Here's how the part is built. I have some questions about the finished solid (model axes, mm). Face numbers are marked on the shaded views. A direction names the side the tool comes from. Coordinates: 2 decimals unless noted, no trailing zeros. Loops run counter-clockwise (first coordinate to the right, second up) from the corner with the lowest first, then second, coordinate; pieces in that order, holes last.
from build123d import *

# Parameters (mm, degrees)
F0_R     = 5
F0_R_2   = 3.15
F0_R_3   = 2.55
F1_DEPTH = 3.25
F2_R     = 2.55
F3_DEPTH = 14


# Not quite as in the source:
# - a feature names something its author has since deleted; it is built from what else it names


with BuildPart() as f1:
    # F0 (on Top) → F1 (new body)
    with BuildSketch(Plane.XY):
        with BuildLine():
            Line((-5.95, -4.4), (-4.4034787385, -4.4))
            ThreePointArc((-4.4034787385, -4.4), (0, -6.225), (4.4034787385, -4.4))
            Line((4.4034787385, -4.4), (5.95, -4.4))
            Line((5.95, -4.4), (5.95, 4.4))
            Line((5.95, 4.4), (4.4034787385, 4.4))
            ThreePointArc((4.4034787385, 4.4), (0, 6.225), (-4.4034787385, 4.4))
            Line((-4.4034787385, 4.4), (-5.95, 4.4))
            Line((-5.95, 4.4), (-5.95, -4.4))
        make_face()
        Circle(F0_R, mode=Mode.SUBTRACT)
        Circle(F0_R)
        Circle(F0_R_2, mode=Mode.SUBTRACT)
        Circle(F0_R_2)
        Circle(F0_R_3, mode=Mode.SUBTRACT)
        Circle(F0_R_3)
        with BuildLine():
            ThreePointArc((-1.275, -0.9666307465), (-0.5099019514, 1.5165750888), (1.6, 0))
            ThreePointArc((1.6, 0), (1.5165750888, -0.5099019514), (1.275, -0.9666307465))
            ThreePointArc((1.275, -0.9666307465), (0, -1.6), (-1.275, -0.9666307465))
        make_face(mode=Mode.SUBTRACT)
        with BuildLine():
            Line((1.275, -0.9666307465), (-1.275, -0.9666307465))
            ThreePointArc((-1.275, -0.9666307465), (0, -1.6), (1.275, -0.9666307465))
        make_face()
    extrude(amount=F1_DEPTH)

    # F2 (on face) → F3 (join)
    with BuildSketch(Plane.XY.offset(3.25)):
        with BuildLine():
            ThreePointArc((-4.8302633262, 0.3000085552), (-4.9546244936, 0.172348246), (-5, 0))
            ThreePointArc((-5, 0), (-4.9546244936, -0.172348246), (-4.8302633262, -0.3000085552))
            Line((-4.8302633262, -0.3000085552), (-4.2601369618, -0.6425750355))
            ThreePointArc((-4.2601369618, -0.6425750355), (-4.0929165173, -0.7205512094), (-3.9131380826, -0.7620563314))
            Line((-3.9131380826, -0.7620563314), (-3.3117988826, -0.835891501))
            ThreePointArc((-3.3117988826, -0.835891501), (-3.0868883315, -0.9291389359), (-2.9422567869, -1.125))
            ThreePointArc((-2.9422567869, -1.125), (-3.15, 0), (-2.9422567869, 1.125))
            ThreePointArc((-2.9422567869, 1.125), (-3.0868883315, 0.9291389359), (-3.3117988826, 0.835891501))
            Line((-3.3117988826, 0.835891501), (-3.9131380826, 0.7620563314))
            ThreePointArc((-3.9131380826, 0.7620563314), (-4.0929165173, 0.7205512094), (-4.2601369618, 0.6425750355))
            Line((-4.2601369618, 0.6425750355), (-4.8302633262, 0.3000085552))
        make_face()
        with BuildLine():
            ThreePointArc((-3.2033738691, 3.6276500367), (-3.3815799641, 3.6253171911), (-3.5355339059, 3.5355339059))
            ThreePointArc((-3.5355339059, 3.5355339059), (-3.6253171911, 3.3815799641), (-3.6276500367, 3.2033738691))
            Line((-3.6276500367, 3.2033738691), (-3.4667408995, 2.5580025694))
            ThreePointArc((-3.4667408995, 2.5580025694), (-3.4036356706, 2.3846223779), (-3.3058616735, 2.2281512744))
            Line((-3.3058616735, 2.2281512744), (-2.9328599965, 1.7507308991))
            ThreePointArc((-2.9328599965, 1.7507308991), (-2.8397601142, 1.5257592297), (-2.8759848548, 1.2849945972))
            ThreePointArc((-2.8759848548, 1.2849945972), (-2.2273863607, 2.2273863607), (-1.2849945972, 2.8759848548))
            ThreePointArc((-1.2849945972, 2.8759848548), (-1.5257592297, 2.8397601142), (-1.7507308991, 2.9328599965))
            Line((-1.7507308991, 2.9328599965), (-2.2281512744, 3.3058616735))
            ThreePointArc((-2.2281512744, 3.3058616735), (-2.3846223779, 3.4036356706), (-2.5580025694, 3.4667408995))
            Line((-2.5580025694, 3.4667408995), (-3.2033738691, 3.6276500367))
        make_face()
        with BuildLine():
            ThreePointArc((0.3000085552, 4.8302633262), (0.172348246, 4.9546244936), (0, 5))
            ThreePointArc((0, 5), (-0.172348246, 4.9546244936), (-0.3000085552, 4.8302633262))
            Line((-0.3000085552, 4.8302633262), (-0.6425750355, 4.2601369618))
            ThreePointArc((-0.6425750355, 4.2601369618), (-0.7205512094, 4.0929165173), (-0.7620563314, 3.9131380826))
            Line((-0.7620563314, 3.9131380826), (-0.835891501, 3.3117988826))
            ThreePointArc((-0.835891501, 3.3117988826), (-0.9291389359, 3.0868883315), (-1.125, 2.9422567869))
            ThreePointArc((-1.125, 2.9422567869), (0, 3.15), (1.125, 2.9422567869))
            ThreePointArc((1.125, 2.9422567869), (0.9291389359, 3.0868883315), (0.835891501, 3.3117988826))
            Line((0.835891501, 3.3117988826), (0.7620563314, 3.9131380826))
            ThreePointArc((0.7620563314, 3.9131380826), (0.7205512094, 4.0929165173), (0.6425750355, 4.2601369618))
            Line((0.6425750355, 4.2601369618), (0.3000085552, 4.8302633262))
        make_face()
        with BuildLine():
            ThreePointArc((3.2033738691, -3.6276500367), (3.3815799667, -3.6253171904), (3.5355339096, -3.5355339023))
            ThreePointArc((3.5355339096, -3.5355339023), (3.6253171918, -3.3815799616), (3.6276500367, -3.2033738691))
            Line((3.6276500367, -3.2033738691), (3.4667408995, -2.5580025694))
            ThreePointArc((3.4667408995, -2.5580025694), (3.4036356706, -2.3846223779), (3.3058616735, -2.2281512744))
            Line((3.3058616735, -2.2281512744), (2.9328599965, -1.7507308991))
            ThreePointArc((2.9328599965, -1.7507308991), (2.8397601142, -1.5257592297), (2.8759848548, -1.2849945972))
            ThreePointArc((2.8759848548, -1.2849945972), (2.2273863607, -2.2273863607), (1.2849945972, -2.8759848548))
            ThreePointArc((1.2849945972, -2.8759848548), (1.5257592297, -2.8397601142), (1.7507308991, -2.9328599965))
            Line((1.7507308991, -2.9328599965), (2.2281512744, -3.3058616735))
            ThreePointArc((2.2281512744, -3.3058616735), (2.3846223779, -3.4036356706), (2.5580025694, -3.4667408995))
            Line((2.5580025694, -3.4667408995), (3.2033738691, -3.6276500367))
        make_face()
        with BuildLine():
            ThreePointArc((-0.3000085552, -4.8302633262), (-0.172348246, -4.9546244936), (0, -5))
            ThreePointArc((0, -5), (0.172348246, -4.9546244936), (0.3000085552, -4.8302633262))
            Line((0.3000085552, -4.8302633262), (0.6425750355, -4.2601369618))
            ThreePointArc((0.6425750355, -4.2601369618), (0.7205512094, -4.0929165173), (0.7620563314, -3.9131380826))
            Line((0.7620563314, -3.9131380826), (0.835891501, -3.3117988826))
            ThreePointArc((0.835891501, -3.3117988826), (0.9291389359, -3.0868883315), (1.125, -2.9422567869))
            ThreePointArc((1.125, -2.9422567869), (0, -3.15), (-1.125, -2.9422567869))
            ThreePointArc((-1.125, -2.9422567869), (-0.9291389359, -3.0868883315), (-0.835891501, -3.3117988826))
            Line((-0.835891501, -3.3117988826), (-0.7620563314, -3.9131380826))
            ThreePointArc((-0.7620563314, -3.9131380826), (-0.7205512094, -4.0929165173), (-0.6425750355, -4.2601369618))
            Line((-0.6425750355, -4.2601369618), (-0.3000085552, -4.8302633262))
        make_face()
        with BuildLine():
            ThreePointArc((-3.6276500367, -3.2033738691), (-3.6253171911, -3.3815799641), (-3.5355339059, -3.5355339059))
            ThreePointArc((-3.5355339059, -3.5355339059), (-3.3815799641, -3.6253171911), (-3.2033738691, -3.6276500367))
            Line((-3.2033738691, -3.6276500367), (-2.5580025694, -3.4667408995))
            ThreePointArc((-2.5580025694, -3.4667408995), (-2.3846223779, -3.4036356706), (-2.2281512744, -3.3058616735))
            Line((-2.2281512744, -3.3058616735), (-1.7507308991, -2.9328599965))
            ThreePointArc((-1.7507308991, -2.9328599965), (-1.5257592297, -2.8397601142), (-1.2849945972, -2.8759848548))
            ThreePointArc((-1.2849945972, -2.8759848548), (-2.2273863607, -2.2273863607), (-2.8759848548, -1.2849945972))
            ThreePointArc((-2.8759848548, -1.2849945972), (-2.8397601142, -1.5257592297), (-2.9328599965, -1.7507308991))
            Line((-2.9328599965, -1.7507308991), (-3.3058616735, -2.2281512744))
            ThreePointArc((-3.3058616735, -2.2281512744), (-3.4036356706, -2.3846223779), (-3.4667408995, -2.5580025694))
            Line((-3.4667408995, -2.5580025694), (-3.6276500367, -3.2033738691))
        make_face()
        with BuildLine():
            ThreePointArc((2.8759848548, -1.2849945972), (2.9102205274, -1.205452812), (2.9422567869, -1.125))
            ThreePointArc((2.9422567869, -1.125), (3.0976288414, -0.5720101054), (3.15, 0))
            ThreePointArc((3.15, 0), (3.0976288414, 0.5720101054), (2.9422567869, 1.125))
            ThreePointArc((2.9422567869, 1.125), (2.9102205274, 1.205452812), (2.8759848548, 1.2849945972))
            ThreePointArc((2.8759848548, 1.2849945972), (2.2273863607, 2.2273863607), (1.2849945972, 2.8759848548))
            ThreePointArc((1.2849945972, 2.8759848548), (1.205452812, 2.9102205274), (1.125, 2.9422567869))
            ThreePointArc((1.125, 2.9422567869), (0, 3.15), (-1.125, 2.9422567869))
            ThreePointArc((-1.125, 2.9422567869), (-1.205452812, 2.9102205274), (-1.2849945972, 2.8759848548))
            ThreePointArc((-1.2849945972, 2.8759848548), (-2.2273863607, 2.2273863607), (-2.8759848548, 1.2849945972))
            ThreePointArc((-2.8759848548, 1.2849945972), (-2.9102205274, 1.205452812), (-2.9422567869, 1.125))
            ThreePointArc((-2.9422567869, 1.125), (-3.15, 0), (-2.9422567869, -1.125))
            ThreePointArc((-2.9422567869, -1.125), (-2.9102205274, -1.205452812), (-2.8759848548, -1.2849945972))
            ThreePointArc((-2.8759848548, -1.2849945972), (-2.2273863607, -2.2273863607), (-1.2849945972, -2.8759848548))
            ThreePointArc((-1.2849945972, -2.8759848548), (-1.205452812, -2.9102205274), (-1.125, -2.9422567869))
            ThreePointArc((-1.125, -2.9422567869), (0, -3.15), (1.125, -2.9422567869))
            ThreePointArc((1.125, -2.9422567869), (1.205452812, -2.9102205274), (1.2849945972, -2.8759848548))
            ThreePointArc((1.2849945972, -2.8759848548), (2.2273863607, -2.2273863607), (2.8759848548, -1.2849945972))
        make_face()
        Circle(F2_R, mode=Mode.SUBTRACT)
        Circle(F2_R)
        with BuildLine():
            ThreePointArc((-1.275, -0.9666307465), (0, 1.6), (1.275, -0.9666307465))
            Line((1.275, -0.9666307465), (-1.275, -0.9666307465))
        make_face(mode=Mode.SUBTRACT)
        with BuildLine():
            ThreePointArc((3.6276500367, 3.2033738691), (3.6253171915, 3.3815799629), (3.5355339078, 3.5355339041))
            ThreePointArc((3.5355339078, 3.5355339041), (3.3815799654, 3.6253171908), (3.2033738691, 3.6276500367))
            Line((3.2033738691, 3.6276500367), (2.5580025694, 3.4667408995))
            ThreePointArc((2.5580025694, 3.4667408995), (2.3846223779, 3.4036356706), (2.2281512744, 3.3058616735))
            Line((2.2281512744, 3.3058616735), (1.7507308991, 2.9328599965))
            ThreePointArc((1.7507308991, 2.9328599965), (1.5257592297, 2.8397601142), (1.2849945972, 2.8759848548))
            ThreePointArc((1.2849945972, 2.8759848548), (2.2273863607, 2.2273863607), (2.8759848548, 1.2849945972))
            ThreePointArc((2.8759848548, 1.2849945972), (2.8397601142, 1.5257592297), (2.9328599965, 1.7507308991))
            Line((2.9328599965, 1.7507308991), (3.3058616735, 2.2281512744))
            ThreePointArc((3.3058616735, 2.2281512744), (3.4036356706, 2.3846223779), (3.4667408995, 2.5580025694))
            Line((3.4667408995, 2.5580025694), (3.6276500367, 3.2033738691))
        make_face()
        with BuildLine():
            ThreePointArc((4.8302633262, -0.3000085552), (4.9546244936, -0.172348246), (5, 0))
            ThreePointArc((5, 0), (4.9546244936, 0.172348246), (4.8302633262, 0.3000085552))
            Line((4.8302633262, 0.3000085552), (4.2601369618, 0.6425750355))
            ThreePointArc((4.2601369618, 0.6425750355), (4.0929165173, 0.7205512094), (3.9131380826, 0.7620563314))
            Line((3.9131380826, 0.7620563314), (3.3117988826, 0.835891501))
            ThreePointArc((3.3117988826, 0.835891501), (3.0868883315, 0.9291389359), (2.9422567869, 1.125))
            ThreePointArc((2.9422567869, 1.125), (3.0976288414, 0.5720101054), (3.15, 0))
            ThreePointArc((3.15, 0), (3.0976288414, -0.5720101054), (2.9422567869, -1.125))
            ThreePointArc((2.9422567869, -1.125), (3.0868883315, -0.9291389359), (3.3117988826, -0.835891501))
            Line((3.3117988826, -0.835891501), (3.9131380826, -0.7620563314))
            ThreePointArc((3.9131380826, -0.7620563314), (4.0929165173, -0.7205512094), (4.2601369618, -0.6425750355))
            Line((4.2601369618, -0.6425750355), (4.8302633262, -0.3000085552))
        make_face()
    extrude(amount=F3_DEPTH)


solid = f1.part
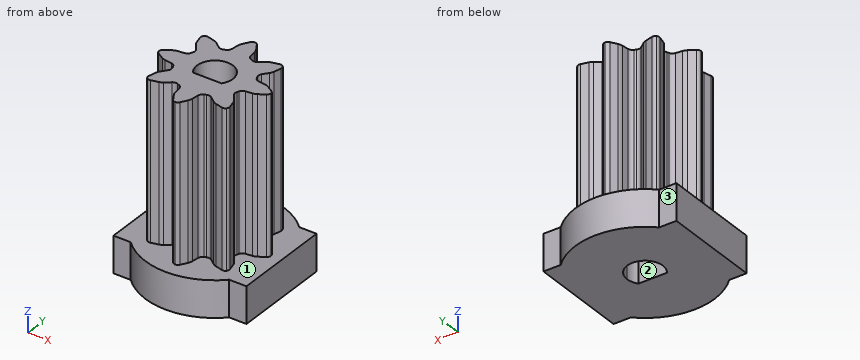
Q1. Please list where these lines run through material, in increasing order: probe 1 along X at (y, z) = (0, 1.45); probe 2 along Y at (x, z) = (0, 2) (3 decimals); probe 3 along Z at (x, y) = (-4.5, -2.75).
Q2. Suppose I cut it at A-A on y = -5.25. Write out the boundary of the cut face in (x, z).
Q3. For the marked faces 1, 2 and 3, which set-ups out of +Z, -Z, +X, -X, +Y, -Y let a thin tool reach every point of the face, with its end or its side?
Q4. Will these pins go through, and if not, where does the flat tip stop? P1, Ø1.5, axis at x = 3, z = 6, coming from the +Y side; P2, Ø4, axis at y = 0.5, z = 8, coming from the -X side; P3, Ø1.2, axis at x = -5.5, z = 1.5, coming from the +Y side.
Check values:
1. probe 1: x = -5.95 to -1.6, 1.6 to 5.95
1. probe 2: y = -6.225 to -0.967, 1.6 to 6.225
1. probe 3: z = 0 to 3.25
2. outline: (-3.34, 0) - (3.34, 0) - (3.34, 3.25) - (-3.34, 3.25) - close
3. face 1: +Z
3. face 2: +Z, -Z
3. face 3: +Z, -Z, -X, +Y
4. P1: stops at y = 3.64
4. P2: stops at x = -5
4. P3: stops at y = 4.4
